Part model, mm, in its own coordinate system. A direction names the side the tool comes from. Give positions to 0.01 mm unless a question says otherwise; leave off trailing zeros. Order: outer loops, then holes, each group sorted by start corner. A loop starts at its lowest first (then second) coordinate and runs counter-clockwise, first axis right, second up. Notation, with made-up numbers: M 3.25,76 L 43.25,76 A22 cw 43.25,91 Z; hole C 46.25,33 d10. An arc over 180 degrees is marked long. One line per question, with ' | ' between items.
```python
from build123d import *

# Parameters (mm, degrees)
SKETCH1_R           = 6
SKETCH1_R_2         = 3.354101966
BOSS_EXTRUDE1_DEPTH = 3


with BuildPart() as part:
    # Sketch1 → Boss-Extrude1 (new body)
    with BuildSketch(Plane(origin=(0, 0, 0), x_dir=(0, 0, -1), z_dir=(1, 0, 0))):
        with Locations((-33.580329287, -7.15217083)):
            Circle(SKETCH1_R)
        with Locations((-33.580329287, -7.15217083)):
            Circle(SKETCH1_R_2, mode=Mode.SUBTRACT)
        with BuildLine():
            Line((-35.080329287, -4.15217083), (-32.080329287, -4.15217083))
            ThreePointArc((-32.080329287, -4.15217083), (-33.580329287, -3.798068864), (-35.080329287, -4.15217083))
        make_face()
        with BuildLine():
            ThreePointArc((-35.080329287, -4.15217083), (-36.934431253, -7.15217083), (-35.080329287, -10.15217083))
            Line((-35.080329287, -10.15217083), (-35.080329287, -4.15217083))
        make_face()
        with BuildLine():
            Line((-32.080329287, -4.15217083), (-32.080329287, -10.15217083))
            ThreePointArc((-32.080329287, -10.15217083), (-30.727159738, -8.915526587), (-30.22622732, -7.15217083))
            ThreePointArc((-30.22622732, -7.15217083), (-30.727159738, -5.388815073), (-32.080329287, -4.15217083))
        make_face()
        with BuildLine():
            ThreePointArc((-35.080329287, -10.15217083), (-33.580329287, -10.506272796), (-32.080329287, -10.15217083))
            Line((-32.080329287, -10.15217083), (-35.080329287, -10.15217083))
        make_face()
    extrude(amount=BOSS_EXTRUDE1_DEPTH)


solid = part.part
```
1. Slice it at B-B on z = 33.25. Give the cut face in (x, y).
Worked out:
outline: M 0,-13.14 L 3,-13.14 L 3,-10.15 L 0,-10.15 Z; M 0,-4.15 L 3,-4.15 L 3,-1.16 L 0,-1.16 Z
2. Mould opens along Y. For faces 1 (the flat face through (1, -10.152, 34)), 2 (the flat face through (0, -7, 31)), 3 (the cylindrical face through (1.479, -6.888, 39.575)) say: released by +Y, released by -Y, zero draft, split by the parting line, or undercut.
Worked out:
face 1: undercut | face 2: zero draft | face 3: split by the parting line
3. Probe L1, parallel to Y at x = 2.3, z = 33.25; L2, parallel to Z at x = 0.4, y = -4.25; L3, parallel to Z at x = 1.35, y = -6. List the from-to ranges inside material, lowest first. Write a range as from..to.
Worked out:
L1: y = -13.14..-10.15, -4.15..-1.16 | L2: z = 28.33..32.08, 35.08..38.83 | L3: z = 27.69..32.08, 35.08..39.47
4. Slice it at A-A on y = -10. Give the cut face in (x, z).
Worked out:
outline: M 0,28.3 L 3,28.3 L 3,32.08 L 0,32.08 Z; M 0,35.08 L 3,35.08 L 3,38.86 L 0,38.86 Z
5. Slice it at C-C on x = 2.2. Give the cut face in (y, z), then the cut area to 3 significant figures.
Worked out:
outline: C -7.15,33.58 d12; hole M -10.15,32.08 L -4.15,32.08 L -4.15,35.08 L -10.15,35.08 Z | area: 95.1 mm2
6. Drop flat-ended pins along their axis: pin 1 (1.5 mm diameter, centred on x = 0.5, y = -4.5, fed in from +Z); pin 2 (1.5 mm diameter, centred on y = -4, z = 37.5, fed in from -X). Give the stop position or say it passes through.
Worked out:
pin 1: stops at z = 39.27 | pin 2: stops at x = 0
7. Tool access for faces 4 (the flat face through (3, -7, 31)), 5 (the flat face through (1, -4.152, 34)): list every direction of +Z, -Z, +X, -X, +Y, -Y with a clear straight run to the whole face (end or side of a thin tool).
Worked out:
face 4: +Z, -Z, +X, +Y, -Y | face 5: +X, -X
8. Slice it at D-D on z = 36. Give the cut face in (x, y).
Worked out:
outline: M 0,-12.64 L 3,-12.64 L 3,-1.66 L 0,-1.66 Z
